```python
from build123d import *

# Parameters (mm, degrees)
EXTRUDE_1_DEPTH         = 2
HOLE_WIZARD_3_2_3_2_1_D = 3.2
HOLE_WIZARD_4_2_4_2_1_D = 4.2
CUT_EXTRUDE_1_DEPTH     = 193.429207762
FILLET_1_R              = 2
FILLET_1_OF_MIRROR_2_R  = 2


with BuildPart() as part:
    # 草图1 → 凸台-拉伸1 (new body)
    with BuildSketch(Plane(origin=(0, 0, 0), x_dir=(0, 0, -1), z_dir=(1, 0, 0))):
        Polygon((-103.494784444, -80), (103.494784444, -80), (175, -20), (175, 0), (-175, 0), (-175, -20), align=None)
    extrude(amount=EXTRUDE_1_DEPTH)

    # Ø3.2 (3.2) 直径孔1 (through all)
    with Locations(Plane(origin=(2, -77, 90), x_dir=(0, 0, 1), z_dir=(1, 0, 0))):
        with Locations((0, 0), (-20, 0), (-180, 0), (-160, 0)):
            Hole(HOLE_WIZARD_3_2_3_2_1_D / 2)

    # Ø4.2 (4.2) 直径孔1 (through all)
    with Locations(Plane(origin=(2, -10, 135), x_dir=(0, 0, 1), z_dir=(1, 0, 0))):
        with Locations((0, 0), (-20, 0), (-65, 0), (-105, 0)):
            hole_wizard_4_2_4_2_1 = Hole(HOLE_WIZARD_4_2_4_2_1_D / 2)

    # 镜向1: Ø4.2 (4.2) 直径孔1 across plane
    add(hole_wizard_4_2_4_2_1.mirror(Plane.XY), mode=Mode.SUBTRACT)

    # 草图6 → 切除-拉伸1 (cut, through all)
    with BuildSketch(Plane(origin=(2, 0, 0), x_dir=(0, 0, -1), z_dir=(1, 0, 0))):
        Polygon((-87.438218406, -20), (-119.551180502, -46.94597465), (-131.996971117, -36.502716336), (-112.329799636, -20), align=None)
        Polygon((-78.103875445, -20), (-114.884009021, -50.862196518), (-102.438218406, -61.305454833), (-53.212294215, -20), align=None)
        Polygon((-44.604098668, -20.609310027), (-56.907628403, -30.93319729), (-22.840825693, -65), (-10, -65), (-10, -55.213408695), align=None)
        Polygon((-151.664142597, -20), (-121.664142597, -20), (-136.664142597, -32.586494468), align=None)
        Polygon((-10, -20), (-10, -46.728127321), (-36.728127321, -20), align=None)
        Polygon((-31.326107067, -65), (-53.953524065, -65), (-73.824981789, -45.128542276), (-61.521452054, -34.804655014), align=None)
        Polygon((-78.438805439, -49), (-62.438805439, -65), (-97.506862921, -65), align=None)
    cut_extrude_1 = extrude(amount=-CUT_EXTRUDE_1_DEPTH, mode=Mode.SUBTRACT)

    # 圆角1
    fillet_1_edges = [part.edges().sort_by_distance(p)[0] for p in [
        (1, -20, 53.212294215),
        (1, -61.305454833, 102.438218406),
        (1, -50.862196518, 114.884009021),
        (1, -20, 78.103875445),
        (1, -36.502716336, 131.996971117),
        (1, -20, 112.329799636),
        (1, -20, 87.438218406),
        (1, -46.94597465, 119.551180502),
        (1, -20, 36.728127321),
        (1, -20, 10),
        (1, -46.728127321, 10),
        (1, -55.213408695, 10),
        (1, -65, 10),
        (1, -65, 22.840825693),
        (1, -30.93319729, 56.907628403),
        (1, -20.609310027, 44.604098668),
        (1, -65, 97.506862921),
        (1, -49, 78.438805439),
        (1, -65, 62.438805439),
        (1, -34.804655014, 61.521452054),
        (1, -65, 31.326107067),
        (1, -65, 53.953524065),
        (1, -45.128542276, 73.824981789),
        (1, -32.586494468, 136.664142597),
        (1, -20, 151.664142597),
        (1, -20, 121.664142597),
    ]]
    fillet(fillet_1_edges, radius=FILLET_1_R)

    # 镜向2: 切除-拉伸1 across plane
    add(cut_extrude_1.mirror(Plane.XY), mode=Mode.SUBTRACT)

    # 圆角1 of 镜向2
    fillet_1_of_mirror_2_edges = [part.edges().sort_by_distance(p)[0] for p in [
        (1, -20, -53.212294215),
        (1, -61.305454833, -102.438218406),
        (1, -50.862196518, -114.884009021),
        (1, -20, -78.103875445),
        (1, -36.502716336, -131.996971117),
        (1, -20, -112.329799636),
        (1, -20, -87.438218406),
        (1, -46.94597465, -119.551180502),
        (1, -20, -36.728127321),
        (1, -20, -10),
        (1, -46.728127321, -10),
        (1, -55.213408695, -10),
        (1, -65, -10),
        (1, -65, -22.840825693),
        (1, -30.93319729, -56.907628403),
        (1, -20.609310027, -44.604098668),
        (1, -65, -97.506862921),
        (1, -49, -78.438805439),
        (1, -65, -62.438805439),
        (1, -34.804655014, -61.521452054),
        (1, -65, -31.326107067),
        (1, -65, -53.953524065),
        (1, -45.128542276, -73.824981789),
        (1, -32.586494468, -136.664142597),
        (1, -20, -151.664142597),
        (1, -20, -121.664142597),
    ]]
    fillet(fillet_1_of_mirror_2_edges, radius=FILLET_1_OF_MIRROR_2_R)


solid = part.part
```
Work out the finished part from the listing and answer in its coordinate system (mm). Round coordinates to 2 decimals unless told otherwise and drop trailing zeros. Write each loop counter-clockwise with the first axis right and the second up, starting at its lowest first coordinate (ties: lowest second). Pieces come first, ordered by that corner, then holes.
1) Consider probe 1 along Y at (x, z) = (0.9, 110.5); probe 2 along Y at (x, z) = (1.2, 41); probe 3 along Y at (x, z) = (1.2, -70). Determine where each line is inside the solid, lowest interval first.
2) A cutting plane is placed at B-B on x = 0.3. Give the number of separate pieces and of enclosed holes in the cut face, and give its area (3 significant figures).
3) A cutting plane is placed at A-A on z = -39.5. Determine the outline of the cut face in (x, y), and give its area (3 significant figures).
4) Flat-ended cylindrical pins translate along their axes: P1, Ø2.5, axis at y = -10, z = 135, coming from the -X side; P2, Ø1, axis at x = 1.5, z = -105.5, coming from the -Y side; P3, Ø0.6, axis at x = 1, y = -61, coming from the -Z side; P4, Ø1, axis at x = 0.5, y = -34.5, coming from the +Z side. Find the tip coordinate at first contact, or state that the pin passes through.
5) Determine the mould class of faces 1 (the face through (2, -39, 2)), 2 (the face through (0.986, -50.42, -138.747)), 3 (the face through (1.014, -25.605, 50.557)), 4 (the face through (1.014, -34.543, -104.77)) for opening direction Y: pulls with the +Y half, pulls with the -Y half, needs draft (parallel to the pull), parting line crosses it, or undercut.
Entries:
1. probe 1: y = -74.12 to -54.54, -47.18 to -39.35, -20 to 0
1. probe 2: y = -80 to -65, -55.33 to -46.84, -24.21 to 0
1. probe 3: y = -80 to -78.6, -75.4 to -65, -57.44 to -48.95, -41.92 to -34.09, -20 to -12.1, -7.9 to 0
2. separate pieces: 1
2. enclosed holes: 26
2. area: 16,300 mm2
3. outline: (0, -80) - (2, -80) - (2, -65) - (0, -65) - close; (0, -56.83) - (2, -56.83) - (2, -48.34) - (0, -48.34) - close; (0, -25.71) - (2, -25.71) - (2, 0) - (0, 0) - close
3. area: 98.4 mm2
4. P1: passes through
4. P2: stops at y = -78.74
4. P3: stops at z = -126.5
4. P4: stops at z = 158.32
5. face 1: needs draft
5. face 2: pulls with the -Y half
5. face 3: undercut
5. face 4: undercut
